```python
from build123d import *

# Parameters (mm, degrees)
SKETCH_1_R            = 10
EXTRUDE_1_DEPTH       = 25
CUT_EXTRUDE_START     = 5
SKETCH_2_W            = 45.854835026
SKETCH_2_H            = 35
SKETCH_2_W_2          = 25.854835026
SKETCH_2_H_2          = 15
CUT_EXTRUDE_2_DEPTH   = 25
SKETCH_3_R            = 3
EXTRUDE_2_DEPTH       = 1.7
SKETCH_4_R            = 1
EXTRUDE_3_DEPTH       = 8
FILLET_1_R            = 2
FILLET_2_R            = 3
SKETCH_5_W            = 5
SKETCH_5_H            = 0.8
EXTRUDE_4_DEPTH       = 2
EXTRUDE_START         = 1
SKETCH_6_R            = 1
EXTRUDE_5_DEPTH       = 1
CUT_EXTRUDE_1_DEPTH   = 6
CUT_EXTRUDE_3_DEPTH   = 0.2
SKETCH_9_W            = 22.189526506
SKETCH_9_H            = 4.332571278
CUT_EXTRUDE_2_2_DEPTH = 5
EXTRUDE_7_DEPTH       = 7
EXTRUDE_7_DEPTH_BACK  = 7
SKETCH_11_W           = 2
SKETCH_11_H           = 0.3
CUT_EXTRUDE_3_2_REACH = 41.498
SKETCH_12_R           = 0.462491299
SKETCH_12_R_2         = 0.396984266


with BuildPart() as part:
    # Эскиз1 → Бобышка-Вытянуть1 (new body)
    with BuildSketch(Plane.XY):
        Circle(SKETCH_1_R)
    extrude(amount=EXTRUDE_1_DEPTH)

    # Эскиз2 → Cut-Extrude 2 (cut)
    with BuildSketch(Plane.XY.offset(CUT_EXTRUDE_START)):
        Rectangle(SKETCH_2_W, SKETCH_2_H)
        Rectangle(SKETCH_2_W_2, SKETCH_2_H_2, mode=Mode.SUBTRACT)
    extrude(amount=CUT_EXTRUDE_2_DEPTH, mode=Mode.SUBTRACT)

    # Эскиз3 → Бобышка-Вытянуть2 (add)
    with BuildSketch(Plane.XY.offset(25)):
        Circle(SKETCH_3_R)
    extrude(amount=EXTRUDE_2_DEPTH)

    # Эскиз4 → Бобышка-Вытянуть3 (add)
    with BuildSketch(Plane.XY.offset(26.7)):
        Circle(SKETCH_4_R)
    extrude(amount=EXTRUDE_3_DEPTH)

    # Скругление1
    fillet_1_edges = [part.edges().sort_by_distance(p)[0] for p in [
        (-10, 0, 25),
        (9.114378278, 4.114378278, 25),
    ]]
    fillet(fillet_1_edges, radius=FILLET_1_R)

    # Скругление2
    fillet_2_edges = [part.edges().sort_by_distance(p)[0] for p in [
        (-10, 0, 0),
    ]]
    fillet(fillet_2_edges, radius=FILLET_2_R)

    # Эскиз5 → Бобышка-Вытянуть4 (add)
    with BuildSketch(Plane(origin=(0, 0, 0), x_dir=(-1, 0, 0), z_dir=(0, 0, -1))):
        with BuildLine():
            Line((-3.570714214, -3.5), (3.570714214, -3.5))
            ThreePointArc((3.570714214, -3.5), (0, 5), (-3.570714214, -3.5))
        make_face()
        with Locations((0, 2.6)):
            Rectangle(SKETCH_5_W, SKETCH_5_H, mode=Mode.SUBTRACT)
    extrude(amount=EXTRUDE_4_DEPTH)

    # Эскиз6 → Бобышка-Вытянуть5 (add)
    with BuildSketch(Plane(origin=(0, 0, -2), x_dir=(-1, 0, 0), z_dir=(0, 0, -1)).offset(EXTRUDE_START)):
        with Locations(Location((0, 0, 0), (0, 0, 180))):
            Circle(SKETCH_6_R)
    extrude(amount=-EXTRUDE_5_DEPTH)

    # Эскиз7 → Вырез-Вытянуть1 (cut)
    with BuildSketch(Plane.XY):
        with BuildLine():
            Line((9.25, 1.6), (12.510793403, 1.6))
            ThreePointArc((12.510793403, 1.6), (14.110793403, 0), (12.510793403, -1.6))
            Line((12.510793403, -1.6), (9.25, -1.6))
            ThreePointArc((9.25, -1.6), (7.65, 0), (9.25, 1.6))
        make_face()
        with BuildLine():
            Line((-9.25, -1.6), (-13.171375323, -1.6))
            ThreePointArc((-13.171375323, -1.6), (-14.771375323, 0), (-13.171375323, 1.6))
            Line((-13.171375323, 1.6), (-9.25, 1.6))
            ThreePointArc((-9.25, 1.6), (-7.65, 0), (-9.25, -1.6))
        make_face()
    extrude(amount=CUT_EXTRUDE_1_DEPTH, mode=Mode.SUBTRACT)

    # Эскиз8 → Cut-Extrude 3 (cut)
    with BuildSketch(Plane.XY.offset(CUT_EXTRUDE_START)):
        with BuildLine():
            Line((6.652067348, -7.6), (-6.652067348, -7.6))
            ThreePointArc((-6.652067348, -7.6), (-10.1, 0), (-6.652067348, 7.6))
            Line((-6.652067348, 7.6), (6.652067348, 7.6))
            ThreePointArc((6.652067348, 7.6), (10.1, 0), (6.652067348, -7.6))
        make_face()
        with BuildLine():
            Line((6.576473219, -7.4), (-6.576473219, -7.4))
            ThreePointArc((-6.576473219, -7.4), (-9.9, 0), (-6.576473219, 7.4))
            Line((-6.576473219, 7.4), (6.576473219, 7.4))
            ThreePointArc((6.576473219, 7.4), (9.9, 0), (6.576473219, -7.4))
        make_face(mode=Mode.SUBTRACT)
    extrude(amount=CUT_EXTRUDE_3_DEPTH, mode=Mode.SUBTRACT)

    # Эскиз9 → Cut-Extrude 2 2 (cut)
    with BuildSketch(Plane.XY):
        with Locations((0.299905464, -9.666285639)):
            Rectangle(SKETCH_9_W, SKETCH_9_H)
        Polygon((4.25, 9), (-4.25, 9), (-4.25, 7.5), (-7.501825295, 7.5), (-7.501825295, 11.857816674), (7.720330833, 11.857816674), (7.720330833, 7.5), (4.25, 7.5), align=None)
    extrude(amount=CUT_EXTRUDE_2_2_DEPTH, mode=Mode.SUBTRACT)

    # Эскиз11 → Бобышка-Вытянуть7 (add, two sides: drawn at the far end of the back side and taken through both)
    with BuildSketch(Plane(origin=(0, 0, 0), x_dir=(0, 0, -1), z_dir=(1, 0, 0)).offset(-EXTRUDE_7_DEPTH_BACK)):
        with Locations((-3, 8.35)):
            Rectangle(SKETCH_11_W, SKETCH_11_H)
    extrude(amount=EXTRUDE_7_DEPTH + EXTRUDE_7_DEPTH_BACK)

    # Эскиз12 → Cut-Extrude 3 2 (cut, up to next)
    with BuildSketch(Plane(origin=(0, 8.5, 0), x_dir=(1, 0, 0), z_dir=(0, 1, 0)), mode=Mode.PRIVATE) as cut_extrude_3_2_sk1:
        with Locations(Location((5.625, -3, 0), (0, 0, 270))):
            Circle(SKETCH_12_R)
    cut_extrude_3_2_tool1 = extrude(cut_extrude_3_2_sk1.sketch, amount=-CUT_EXTRUDE_3_2_REACH, mode=Mode.PRIVATE) & part.part
    # Эскиз12 → Cut-Extrude 3 2 (cut, up to next)
    with BuildSketch(Plane(origin=(0, 8.5, 0), x_dir=(1, 0, 0), z_dir=(0, 1, 0)), mode=Mode.PRIVATE) as cut_extrude_3_2_sk2:
        with Locations(Location((-5.625, -3, 0), (0, 0, 270))):
            Circle(SKETCH_12_R_2)
    cut_extrude_3_2_tool2 = extrude(cut_extrude_3_2_sk2.sketch, amount=-CUT_EXTRUDE_3_2_REACH, mode=Mode.PRIVATE) & part.part
    add(cut_extrude_3_2_tool1.solids().sort_by_distance((5.625, 8.5, 3))[0], mode=Mode.SUBTRACT)
    add(cut_extrude_3_2_tool2.solids().sort_by_distance((-5.625, 8.5, 3))[0], mode=Mode.SUBTRACT)


solid = part.part
```
Can you work these out from the model? Positions are in its coordinate system, mm. A direction names the side the tool comes from. Coordinates: 2 decimals unless noted, no trailing zeros. Loops run counter-clockwise (first coordinate to the right, second up) from the corner with the lowest first, then second, coordinate; pieces in that order, holes last. Notation, with made-up numbers: (-13.5, -25.75) -> (28.5, -25.75) arc R31 cw to (28.5, 1.25) -> close; hole circle Ø9 at (-38, 39). An arc over 180 degrees is marked (long way). Answer as a JSON object with one key per item and string values.
1) For P1, Ø6.5, axis at x = -1, y = -5.5, coming from the +Z side; P2, Ø3, axis at x = 1, z = 14, coming from the +Y side; P3, Ø2, axis at x = -6, z = 3.5, coming from the +Y side, each with a flat end and sliding along its axis, tell me the tip position at first contact or that it passes through.
Results:
{"P1": "stops at z = 26.7", "P2": "stops at y = 7.5", "P3": "stops at y = 8.5"}
2) Thinking about a two-plate mould opening in Y: for faces 5 (the face through (5, 7.5, 3)), 6 (the face through (-0.1, 3.4, 25)), 7 (the face through (-0.217, 0.976, -2.507)), which applies, pulls with the +Y half, pulls with the -Y half, needs draft (parallel to the pull), parting line crosses it, or undercut?
Results:
{"face 5": "undercut", "face 6": "needs draft", "face 7": "parting line crosses it"}
3) For faces 1 (the face through (-5.9, 8.2, 3.5)), 2 (the face through (-8.78, -4.79, 3.99)), 3 (the face through (0, -5, 0)), 4 (the face through (-7.65, 0.04, 2.99)), which set-ups out of +Z, -Z, +X, -X, +Y, -Y let a thin tool reach every point of the face, with its end or its side?
Results:
{"face 1": "+Z, -Z, -X", "face 2": "+Z, -Z, -X, -Y", "face 3": "-Z", "face 4": "-Z, -X"}
4) Imagine slicing it at C-C (z = 19). Please give me the cut outline in (x, y), then the cut area to 3 significant figures.
Results:
{"outline": "(-6.61, -7.5) -> (6.61, -7.5) arc R10 ccw to (6.61, 7.5) -> (-6.61, 7.5) arc R10 ccw to start", "area": "269 mm^2"}
5) Imagine slicing it at D-D (z = 23.5). Please give me the cut outline in (x, y), then the cut area to 3 significant figures.
Results:
{"outline": "(-6.52, -7.5) -> (6.52, -7.5) arc R9.94 ccw to (6.52, 7.5) -> (-6.52, 7.5) arc R9.94 ccw to start", "area": "267 mm^2"}
6) Imagine slicing it at A-A (z = -0.5). Please give me the cut outline in (x, y).
Results:
{"outline": "(-3.57, -3.5) -> (3.57, -3.5) arc R5 ccw (long way) to start; hole (-2.5, 2.2) -> (2.5, 2.2) -> (2.5, 3) -> (-2.5, 3) -> close"}
7) If I drill on line 1 (X direction, y = 8.4, z = 3); line 2 (Z direction, x = -5.5, y = -5); line 3 (Y direction, x = 1.5, z = 18.5), over which ranges is the centre line in solid material (lowest first)?
Results:
{"line 1": "x = -7 to -6.02, -5.23 to 5.16, 6.09 to 7", "line 2": "z = 0.03 to 25", "line 3": "y = -7.5 to 7.5"}
